Work out the finished part from the listing and answer in its coordinate system (mm). Coordinates: 2 decimals unless noted, no trailing zeros. Loops run counter-clockwise (first coordinate to the right, second up) from the corner with the lowest first, then second, coordinate; pieces in that order, holes last. Notation, with made-up numbers: (-6.75, -24.75) -> (5.25, -24.75) arc R21 ccw to (5.25, -15.75) -> close; hole circle Ø3 at (-19.5, 33.25). An arc over 180 degrees is marked (long way). One line per question, with ' | ' between items.
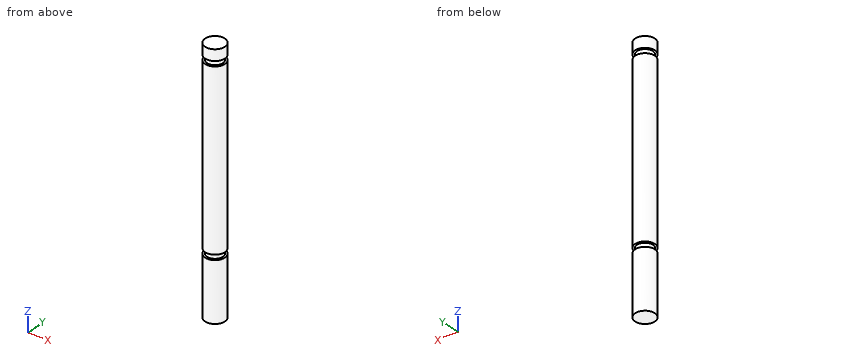
```python
from build123d import *

# Parameters (mm, degrees)
SKETCH2_R           = 3.175
BOSS_EXTRUDE1_DEPTH = 81.28
SKETCH3_OUTSIDE_W   = 24.704
SKETCH3_OUTSIDE_H   = 24.704
SKETCH3_OUTSIDE_R   = 2.54
CUT_EXTRUDE1_DEPTH  = 1.6002
SKETCH4_OUTSIDE_W   = 24.704
SKETCH4_OUTSIDE_H   = 24.704
SKETCH4_OUTSIDE_R   = 2.54
CUT_EXTRUDE2_DEPTH  = 1.6002


with BuildPart() as part:
    # Sketch2 → Boss-Extrude1 (new body)
    with BuildSketch(Plane.XY):
        Circle(SKETCH2_R)
    extrude(amount=BOSS_EXTRUDE1_DEPTH)

    # Sketch3 outside → Cut-Extrude1 (cut)
    with BuildSketch(Plane(origin=(0, 0, 20.4978), x_dir=(-1, 0, 0), z_dir=(0, 0, -1))):
        Rectangle(SKETCH3_OUTSIDE_W, SKETCH3_OUTSIDE_H)
        Circle(SKETCH3_OUTSIDE_R, mode=Mode.SUBTRACT)
    extrude(amount=CUT_EXTRUDE1_DEPTH, mode=Mode.SUBTRACT)

    # Sketch4 outside → Cut-Extrude2 (cut)
    with BuildSketch(Plane.XY.offset(76.2)):
        Rectangle(SKETCH4_OUTSIDE_W, SKETCH4_OUTSIDE_H)
        Circle(SKETCH4_OUTSIDE_R, mode=Mode.SUBTRACT)
    extrude(amount=CUT_EXTRUDE2_DEPTH, mode=Mode.SUBTRACT)


solid = part.part
```
1) Flat-ended cylindrical pins translate along their axes: pin 1 (3 mm diameter, centred on y = 2, z = 15, fed in from +X); pin 2 (2 mm diameter, centred on y = 1, z = 53.5, fed in from +X) (3 decimals). Find the tip coordinate at first contact, or state that the pin passes through.
Check values:
pin 1: stops at x = 3.14 | pin 2: stops at x = 3.175
2) Find section C-C (z = 25). Write down the section's boundary in (x, y) (3 decimals).
Check values:
outline: circle Ø6.35 at (0, 0)
3) Find section B-B (y = 1.5). Write down the section's boundary in (x, z), plus the area to 3 significant figures.
Check values:
outline: (-2.8, 0) -> (2.8, 0) -> (2.8, 18.9) -> (2.05, 18.9) -> (2.05, 20.5) -> (2.8, 20.5) -> (2.8, 76.2) -> (2.05, 76.2) -> (2.05, 77.8) -> (2.8, 77.8) -> (2.8, 81.28) -> (-2.8, 81.28) -> (-2.8, 77.8) -> (-2.05, 77.8) -> (-2.05, 76.2) -> (-2.8, 76.2) -> (-2.8, 20.5) -> (-2.05, 20.5) -> (-2.05, 18.9) -> (-2.8, 18.9) -> close | area: 450 mm^2
4) Find section A-A (x = -0.5). Write down the section's boundary in (y, z), plus the area to 3 significant figures.
Check values:
outline: (-3.14, 0) -> (3.14, 0) -> (3.14, 18.9) -> (2.49, 18.9) -> (2.49, 20.5) -> (3.14, 20.5) -> (3.14, 76.2) -> (2.49, 76.2) -> (2.49, 77.8) -> (3.14, 77.8) -> (3.14, 81.28) -> (-3.14, 81.28) -> (-3.14, 77.8) -> (-2.49, 77.8) -> (-2.49, 76.2) -> (-3.14, 76.2) -> (-3.14, 20.5) -> (-2.49, 20.5) -> (-2.49, 18.9) -> (-3.14, 18.9) -> close | area: 506 mm^2
5) Find the intervals of material crossed by line 1 along Z through (x, y) = (2.5, 1); line 2 along Y through (x, z) = (0.25, 50.5); line 3 along Y through (x, z) = (1.75, 15), in increasing order.
Check values:
line 1: z = 0 to 18.9, 20.5 to 76.2, 77.8 to 81.28 | line 2: y = -3.17 to 3.17 | line 3: y = -2.65 to 2.65
